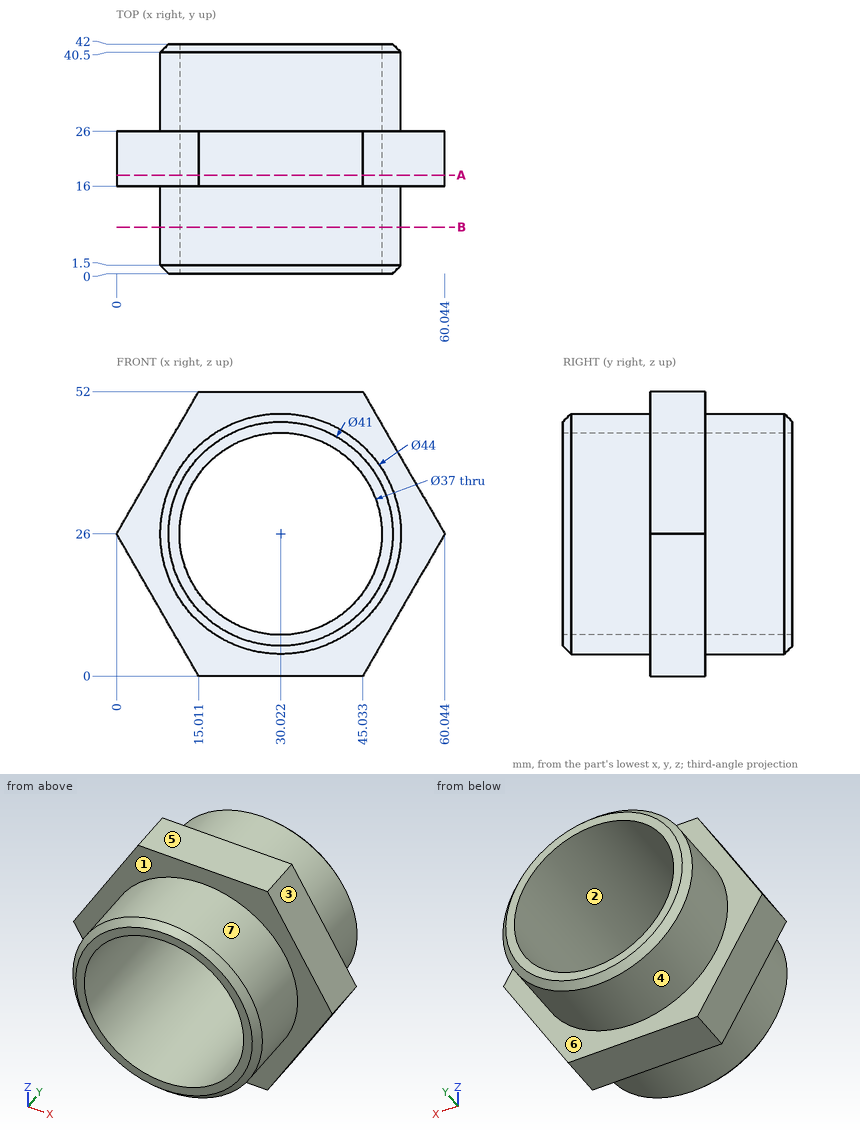
Check sheet for the drawn part. Datum: minimum x, y, z corner. Units: mm. A direction names the side the tool comes from. Round coordinates to 2 decimals unless told otherwise and drop trailing zeros. Write each loop counter-clockwise with the first axis right and the second up, starting at its lowest first coordinate (ties: lowest second). Pieces come first, ordered by that corner, then holes. Notation, with made-up numbers: (80, 64) -> (101, 64) arc R12 cw to (101, 84) -> close; hole circle Ø7 at (-35, 46.25). An arc over 180 degrees is marked (long way). Write each question's results on one line, items separated by ' | '.
Q1. Access from +Z, -Z, +X, -X, +Y, -Y to the whole of each face (thin tool, end or side, straight path). Record for the marked faces 5, 6 and 7.
Derived:
face 5: +Z, +X, -X, +Y, -Y | face 6: +Y | face 7: -Y
Q2. Sectioned sample at A-A, the plane y = 18. Record the boundary of the cut face in (x, z) (1 decimal), and give its area (3 significant figures).
Derived:
outline: (0, 26) -> (15, 0) -> (45, 0) -> (60, 26) -> (45, 52) -> (15, 52) -> close; hole circle Ø37 at (30, 26) | area: 1,270 mm²
Q3. Draft check along Z on the marked faces 1, 2, 3 and 4. Enter one of: released by +Z, released by -Z, zero draft, split by the parting line, or undercut.
Derived:
face 1: zero draft | face 2: undercut | face 3: released by +Z | face 4: split by the parting line
Q4. Go/stop test with flat-tipped pins: pin 1 Ø5 at (y, z) = (22.5, 39.5) entering from -X; pin 2 Ø5 at (x, y) = (45.5, 36) entering from +Z (1 decimal); pin 3 Ø1.5 at (y, z) = (24, 7.5) entering from +X. Record where each tip stops, or that it passes through.
Derived:
pin 1: stops at x = 6.35 | pin 2: stops at z = 43.8 | pin 3: stops at x = 49.8
Q5. Thickness scan on probe 1 along X at (y, z) = (30, 26); probe 2 along Z at (x, y) = (29.5, 40.5) (1 decimal); probe 3 along Z at (x, y) = (38, 32.5). Record the ranges inside material, lowest first.
Derived:
probe 1: x = 8.02 to 11.52, 48.52 to 52.02 | probe 2: z = 4 to 7.5, 44.5 to 48 | probe 3: z = 5.5 to 9.31, 42.69 to 46.5
Q6. Sectioned sample at B-B, the plane y = 8.5. Record the boundary of the cut face in (x, z).
Derived:
outline: circle Ø44 at (30.02, 26); hole circle Ø37 at (30.02, 26)
